from build123d import *

# Parameters (mm, degrees)
SKETCH1_W           = 80
SKETCH1_H           = 70
SKETCH1_R           = 1.5
SKETCH1_R_2         = 2
SKETCH1_R_3         = 4.125
SKETCH1_R_4         = 3
BOSS_EXTRUDE4_DEPTH = 4
SKETCH1_7_R         = 4.5
CUT_EXTRUDE2_DEPTH  = 2


with BuildPart() as part:
    # Sketch1 → Boss-Extrude4 (new body)
    with BuildSketch(Plane(origin=(0, 0, 0), x_dir=(1, 0, 0), z_dir=(0, 1, 0))):
        Rectangle(SKETCH1_W, SKETCH1_H)
        with Locations((-25, 25)):
            Circle(SKETCH1_R, mode=Mode.SUBTRACT)
        with Locations((25, 25)):
            Circle(SKETCH1_R, mode=Mode.SUBTRACT)
        with Locations((25, -24.60667729)):
            Circle(SKETCH1_R, mode=Mode.SUBTRACT)
        with Locations((-25, -24.60667729)):
            Circle(SKETCH1_R, mode=Mode.SUBTRACT)
        with Locations((-3.5, -7.102660735)):
            Circle(SKETCH1_R_2, mode=Mode.SUBTRACT)
        with Locations((31.5, -7.102660735)):
            Circle(SKETCH1_R_2, mode=Mode.SUBTRACT)
        with Locations((-16, 1)):
            Circle(SKETCH1_R_3, mode=Mode.SUBTRACT)
        with Locations((13.978339488, 0.999882702)):
            Circle(SKETCH1_R_4, mode=Mode.SUBTRACT)
    extrude(amount=BOSS_EXTRUDE4_DEPTH)

    # Sketch1<7> → Cut-Extrude2 (cut)
    with BuildSketch(Plane(origin=(0, 0, 0), x_dir=(1, 0, 0), z_dir=(0, 1, 0))):
        with Locations((13.978339488, 0.999882702)):
            Circle(SKETCH1_7_R)
    extrude(amount=CUT_EXTRUDE2_DEPTH, mode=Mode.SUBTRACT)


solid = part.part
For this review, take the finished solid that the model builds, in its own axes (mm). A direction names the side the tool comes from. Give positions to 0.01 mm unless a question says otherwise; leave off trailing zeros. Loops run counter-clockwise (first coordinate to the right, second up) from the corner with the lowest first, then second, coordinate; pieces in that order, holes last. Notation, with made-up numbers: M 82,-37.5 L 91,-37.5 A16 cw 91,-8.5 Z; hole C -1,5.25 d1. An arc over 180 degrees is marked long. Put each result on its own line as item: value. Start each with the question number.
(1) The part is to be moulded in two halves that separate along X. For faces 1 (the flat face through (-40, 2, 0)), 2 (the flat face through (-1, 4, 0)), 3 (the cylindrical face through (-3.76, 1.97, 5.12)), say which applies: +X half, -X half, draft (parallel to the pull), parting line (faces both ways), or undercut.
(2) Add section A-A, the plane x = 25. Write out the cut boundary in (y, z).
(3) Add section B-B, the plane z = -25. Write out the cut boundary in (x, y).
(4) Add section D-D, the plane x = 14.5. Write out the cut boundary in (y, z), then the cut area to 3 significant figures.
(5) For pin 1 (4.5 mm diameter, centred on x = 14.5, z = -3, fed in from -Y), flat-tipped, find the tip position at first contact; note if it passes through.
(6) Add section C-C, the plane y = 1. Give the number of separate pieces and of enclosed holes in the cut face, then the cut area to 3 significant figures.
(7) Wall thickness on L1, parallel to Z at x = -25, y = 1.1; L2, parallel to X at y = 2.9, z = 8; L3, parallel to Z at x = 14, y = 2.5: over which ranges is each line inside the solid? List them lowest first.
(8) Machinability: for faces 4 (the flat face through (15, 2, 2)), 5 (the cylindrical face through (33.408, 1.972, 6.502)), which of the approach directions +Z, -Z, +X, -X, +Y, -Y give a long, thin tool a straight path to every point of the face, cutting with its end or side? Answer none if there is none.
Result:
1. face 1: -X half
1. face 2: draft
1. face 3: undercut
2. outline: M 0,-35 L 4,-35 L 4,-26.5 L 0,-26.5 Z; M 0,-23.5 L 4,-23.5 L 4,23.11 L 0,23.11 Z; M 0,26.11 L 4,26.11 L 4,35 L 0,35 Z
3. outline: M -40,0 L -26.5,0 L -26.5,4 L -40,4 Z; M -23.5,0 L 23.5,0 L 23.5,4 L -23.5,4 Z; M 26.5,0 L 40,0 L 40,4 L 26.5,4 Z
4. outline: M 0,-35 L 4,-35 L 4,-3.95 L 2,-3.95 L 2,-5.47 L 0,-5.47 Z; M 0,3.47 L 2,3.47 L 2,1.95 L 4,1.95 L 4,35 L 0,35 Z
4. area: 250 mm^2
5. pin 1: stops at y = 2
6. separate pieces: 1
6. enclosed holes: 8
6. area: 5,430 mm^2
7. L1: z = -35 to -26.5, -23.5 to 23.11, 26.11 to 35
7. L2: x = -40 to -5.29, -1.71 to 29.71, 33.29 to 40
7. L3: z = -35 to -4, 2 to 35
8. face 4: -Y
8. face 5: +Y, -Y
